Input: part model. Units: mm. Frame: model coordinates. A direction names the side the tool comes from. Round coordinates to 2 decimals unless told otherwise and drop trailing zeros. Order: outer loops, then holes, each group sorted by start corner. A loop starts at its lowest first (then second) coordinate and runs counter-clockwise, first axis right, second up. Notation, with made-up numbers: (30.5, 58) -> (79.5, 58) arc R33 ccw to (79.5, 94) -> close; hole circle Ø10 at (47, -1). An arc over 180 degrees is marked (long way). Use a Markdown table: item, result.
from build123d import *

# Parameters (mm, degrees)
SKETCH1_R               = 8
BOSS_EXTRUDE1_DEPTH     = 20
SKETCH2_R               = 20
BOSS_EXTRUDE2_DEPTH     = 139
SKETCH3_R               = 15
CUT_EXTRUDE1_DEPTH      = 42
CUT_EXTRUDE1_DEPTH_BACK = 57
SKETCH4_W               = 4
SKETCH4_H               = 2.5
SKETCH5_R               = 16
CUT_EXTRUDE2_DEPTH      = 35.4
SKETCH6_R               = 9.5
CUT_EXTRUDE3_DEPTH      = 22
CHAMFER1_SIZE           = 2
FILLET1_R               = 3


with BuildPart() as part:
    # Sketch1 → Boss-Extrude1 (new body)
    with BuildSketch(Plane.XY):
        with BuildLine():
            Line((-56, 40), (41, 40))
            Line((41, 40), (41, 8))
            ThreePointArc((41, 8), (33, 0), (41, -8))
            Line((41, -8), (41, -30))
            Line((41, -30), (-56, -30))
            Line((-56, -30), (-56, 40))
        make_face()
        with Locations((-41, 0)):
            Circle(SKETCH1_R, mode=Mode.SUBTRACT)
    extrude(amount=BOSS_EXTRUDE1_DEPTH)

    # Sketch2 → Boss-Extrude2 (add)
    with BuildSketch(Plane.XY.offset(20)):
        Circle(SKETCH2_R)
    extrude(amount=BOSS_EXTRUDE2_DEPTH)

    # Sketch3 → Cut-Extrude1 (cut, two sides)
    with BuildSketch(Plane(origin=(0, 0, 0), x_dir=(0, 0, -1), z_dir=(1, 0, 0))) as cut_extrude1_sk:
        with Locations((-90, 0)):
            Circle(SKETCH3_R)
    extrude(amount=CUT_EXTRUDE1_DEPTH, mode=Mode.SUBTRACT)
    extrude(cut_extrude1_sk.sketch, amount=-CUT_EXTRUDE1_DEPTH_BACK, mode=Mode.SUBTRACT)

    # Sketch4 → Cut-Revolve1 (revolve, cut)
    with BuildSketch(Plane(origin=(0, 0, 0), x_dir=(0, 0, -1), z_dir=(1, 0, 0))):
        with Locations((-64, 18.75)):
            Rectangle(SKETCH4_W, SKETCH4_H)
        with Locations((-72, 18.75)):
            Rectangle(SKETCH4_W, SKETCH4_H)
        with Locations((-118.6, 18.75)):
            Rectangle(SKETCH4_W, SKETCH4_H)
    revolve(axis=Axis((0, 0, 0), (0, 0, 1)), mode=Mode.SUBTRACT)

    # Sketch5 → Cut-Extrude2 (cut)
    with BuildSketch(Plane.XY.offset(159)):
        Circle(SKETCH5_R)
    extrude(amount=-CUT_EXTRUDE2_DEPTH, mode=Mode.SUBTRACT)

    # Sketch6 → Cut-Extrude3 (cut)
    with BuildSketch(Plane.XY.offset(123.6)):
        Circle(SKETCH6_R)
    extrude(amount=-CUT_EXTRUDE3_DEPTH, mode=Mode.SUBTRACT)

    # Chamfer1
    chamfer1_edges = [part.edges().sort_by_distance(p)[0] for p in [
        (-20, 0, 159),
    ]]
    chamfer(chamfer1_edges, length=CHAMFER1_SIZE)

    # Fillet1
    fillet1_edges = [part.edges().sort_by_distance(p)[0] for p in [
        (-56, 40, 10),
        (-56, -30, 10),
        (-7.5, 40, 0),
        (-7.5, -30, 0),
    ]]
    fillet(fillet1_edges, radius=FILLET1_R)


solid = part.part
1) Line query: L1, parallel to Y at x = 0, z = 138; L2, parallel to X at y = 0, z = 115; L3, parallel to Z at x = -44.5, y = 22.5. Output: solid intervals per line, ascending. Write a range as [from, to].
Results found:
| item | result |
|---|---|
| L1 | y = [-20, -16], [16, 20] |
| L2 | x = [-20, -9.5], [9.5, 20] |
| L3 | z = [0, 20] |
2) Set-up query: faces 1 (the cylindrical face through (-8.18, -29.14, 0.9)), 2 (the flat face through (18, 0, 74)), 3 (the cylindrical face through (18.475, -7.66, 40.706)). Return all of +Z, -Z, +X, -X, +Y, -Y with unobstructed straight access to the full face (end or side cutting, diameter ignored); none if empty.
Results found:
| item | result |
|---|---|
| face 1 | -Z, +X, -X, -Y |
| face 2 | none |
| face 3 | +Z |
3) Cut plane D-D on x = -30.5. Return loops of the section in (y, z), and give its area (3 significant figures).
Results found:
| item | result |
|---|---|
| outline | (-30, 3) arc R3 ccw to (-27, 0) -> (37, 0) arc R3 ccw to (40, 3) -> (40, 20) -> (-30, 20) -> close |
| area | 1,400 mm² |
4) Pin query (flat end, axial travel): pin 1 Ø18.5 at (x, y) = (-41, 0) entering from +Z; pin 2 Ø20 at (x, y) = (3, -1.5) entering from +Z; pin 3 Ø8 at (x, z) = (17.5, 102) entering from +Y. Return the tip coordinate at first contact, or that it passes through.
Results found:
| item | result |
|---|---|
| pin 1 | stops at z = 20 |
| pin 2 | stops at z = 123.6 |
| pin 3 | stops at y = 14.76 |
5) Pull-direction query (X, two-part tool) for faces 4 (the cylindrical face through (-47.349, -4.868, 9.86)), 5 (the cylindrical face through (18.475, -7.66, 67.972)), 6 (the flat face through (41, -19, 10)); classes: +X half, -X half, draft (parallel to the pull), parting line (faces both ways), or undercut.
Results found:
| item | result |
|---|---|
| face 4 | undercut |
| face 5 | parting line |
| face 6 | +X half |
6) Cut plane C-C on z = 149.5. Return loops of the section in (x, y), and give its area (3 significant figures).
Results found:
| item | result |
|---|---|
| outline | circle Ø40 at (0, 0); hole circle Ø32 at (0, 0) |
| area | 452 mm² |
7) Cut plane B-B on y = 0. Count the separate pieces of the cut face and the enclosed holes in it, and give its area (3 significant figures).
Results found:
| item | result |
|---|---|
| separate pieces | 4 |
| enclosed holes | 0 |
| area | 4,270 mm² |
8) Cut plane A-A on x = -41. Return loops of the section in (y, z).
Results found:
| item | result |
|---|---|
| outline | (-30, 3) arc R3 ccw to (-27, 0) -> (-8, 0) -> (-8, 20) -> (-30, 20) -> close; (8, 0) -> (37, 0) arc R3 ccw to (40, 3) -> (40, 20) -> (8, 20) -> close |
